Answer from the drawing. Dimensions are ordinates in mm from the lowest x, y and z of the part. Coordinates: 2 decimals unless noted, no trailing zeros. Write each loop counter-clockwise with the first axis right and the second up, starting at its lowest first coordinate (ties: lowest second). Pieces come first, ordered by that corner, then holes. Notation, with made-up numbers: (-7, -0.75) - (38, -0.75) arc R28 cw to (38, 28.25) - close; hole circle Ø9 at (3.5, -30). An arc over 180 degrees is marked (long way). Use one line per item in the form item = value. Start each with the question number.
Item 1: A cutting plane is placed at A-A (x = 5.5). Write down the section's boundary in (y, z) (1 decimal), then the cut area to 3 significant figures.
Item 2: Determine the mould class of the marked faces 1, 2 and 3 for opening direction Y: released by +Y, released by -Y, zero draft, split by the parting line, or undercut.
Item 3: Given pin 1 (1 mm diameter, centred on y = 2, z = 3.5, fed in from -X); pin 2 (4 mm diameter, centred on x = 3.57, y = 3.57, fed in from -Z); pin 3 (3 mm diameter, centred on y = 2, z = 12.5, fed in from -X) (1 decimal); pin 4 (1 mm diameter, centred on y = 6, z = 19, fed in from +X), each flat-ended and moving along its own axis, determine where each tip first touches the part or whether it passes through.
Item 4: A cutting plane is placed at C-C (z = 3.75). Write down the section's boundary in (x, y) (1 decimal).
Item 5: A cutting plane is placed at D-D (x = 4.25). Write down the section's boundary in (y, z) (1 decimal).
Item 6: Consider probe 1 along Y at (x, z) = (3.5, 12) (1 decimal); probe 2 along Y at (x, z) = (4.75, 9) (1 decimal). Determine where each line is inside the solid, lowest interval first.
Item 7: A cutting plane is placed at B-B (y = 3.25). Write down the section's boundary in (x, z) (1 decimal).
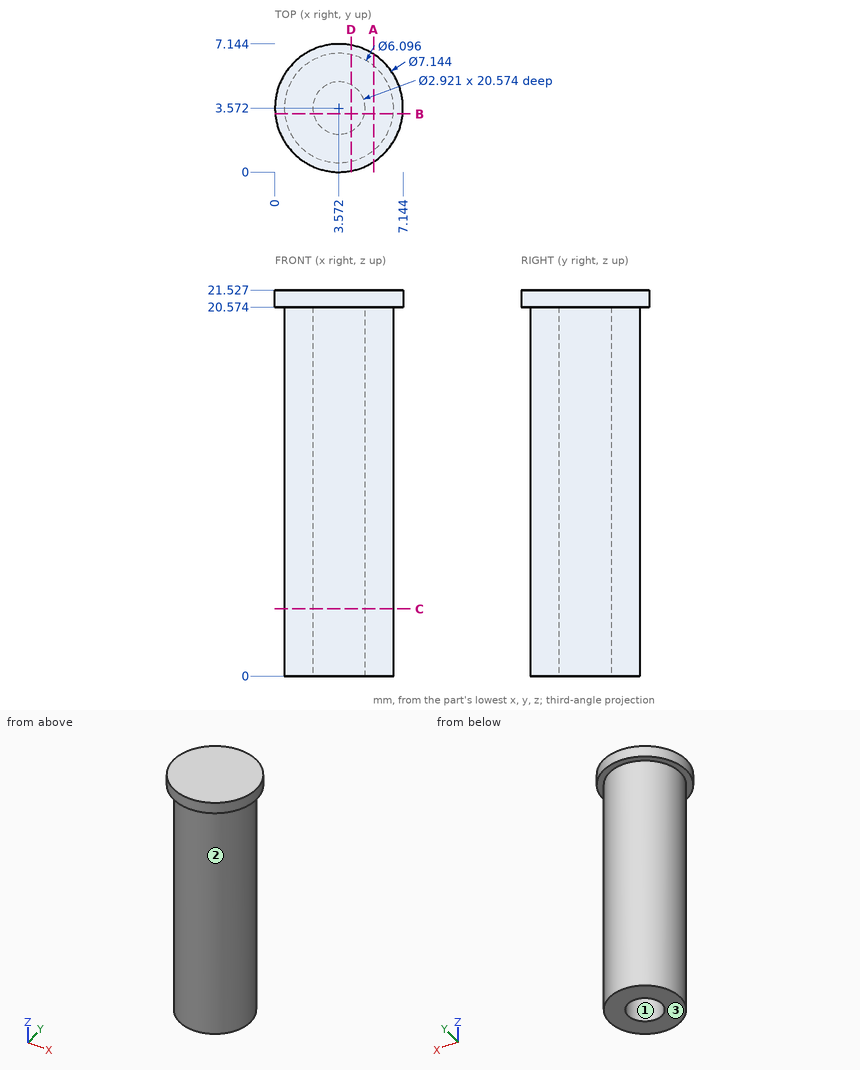
Answer:
q1.outline = (0.6, 20.6) - (1.2, 20.6) - (1.2, 0) - (5.9, 0) - (5.9, 20.6) - (6.6, 20.6) - (6.6, 21.5) - (0.6, 21.5) - close
q1.area = 103 mm²
q2.face_1 = undercut
q2.face_2 = split by the parting line
q2.face_3 = zero draft
q3.pin_1 = 0.72
q3.pin_2 = 0
q3.pin_3 = 0.5
q3.pin_4 = 5.93
q4.outline = circle Ø6.1 at (3.6, 3.6); hole circle Ø2.9 at (3.6, 3.6)
q5.outline = (0.1, 20.6) - (0.6, 20.6) - (0.6, 0) - (2.3, 0) - (2.3, 20.6) - (4.9, 20.6) - (4.9, 0) - (6.5, 0) - (6.5, 20.6) - (7.1, 20.6) - (7.1, 21.5) - (0.1, 21.5) - close
q6.probe_1 = 0.5 to 2.1, 5 to 6.6
q6.probe_2 = 0.8 to 2.7, 4.4 to 6.4
q7.outline = (0, 20.6) - (0.5, 20.6) - (0.5, 0) - (2.1, 0) - (2.1, 20.6) - (5, 20.6) - (5, 0) - (6.6, 0) - (6.6, 20.6) - (7.1, 20.6) - (7.1, 21.5) - (0, 21.5) - close
